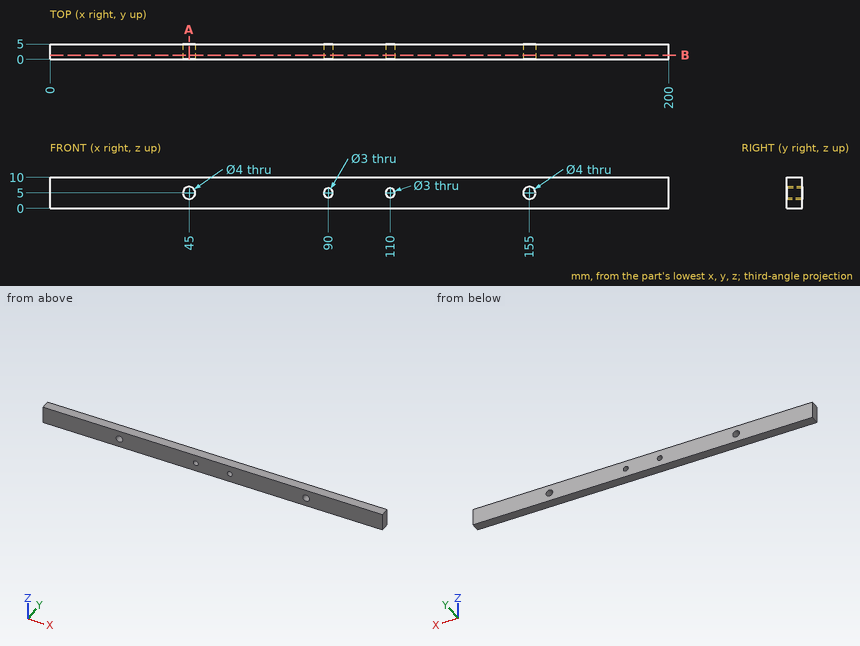
Print and shaded views of the part. All mm, measured from the part's lowest x, y and z. Give positions to 0.01 mm unless a question says otherwise; leave off trailing zeros. Write each loop counter-clockwise with the first axis right and the second up, starting at its lowest first coordinate (ties: lowest second). Pieces come first, ordered by that corner, then holes. Notation, with made-up numbers: M 57,-6 L 104,-6 A12 ccw 104,-2 Z; hole C -10.75,18.25 d9. An arc over 180 degrees is marked long. Use a Markdown table: item, result.
1) Cut at A-A (x = 45). List the corners of the cut face in (y, z), and give its area (3 significant figures).
Responses:
| item | result |
|---|---|
| outline | M 0,0 L 5,0 L 5,3 L 0,3 Z; M 0,7 L 5,7 L 5,10 L 0,10 Z |
| area | 30.0 mm2 |
2) Cut at B-B (y = 1.4). List the corners of the cut face in (x, z), and give its area (3 significant figures).
Responses:
| item | result |
|---|---|
| outline | M 0,0 L 200,0 L 200,10 L 0,10 Z; hole C 45,5 d4; hole C 90,5 d3; hole C 110,5 d3; hole C 155,5 d4 |
| area | 1,960 mm2 |
3) Drill centre lines: line 1 (X direction, y = 3.3, z = 5); line 2 (Z direction, x = 110, y = 1.3); line 3 (Z direction, x = 155, y = 1.2). Where is each one in solid material? Low to high. Write a range as from..to.
Responses:
| item | result |
|---|---|
| line 1 | x = 0..43, 47..88.5, 91.5..108.5, 111.5..153, 157..200 |
| line 2 | z = 0..3.5, 6.5..10 |
| line 3 | z = 0..3, 7..10 |
4) Pin check, flat tip, straight feed: pin 1 (3.5 mm diameter, centred on x = 155, z = 5, fed in from -Y). Stop position of the tip, or through.
Responses:
| item | result |
|---|---|
| pin 1 | passes through |
